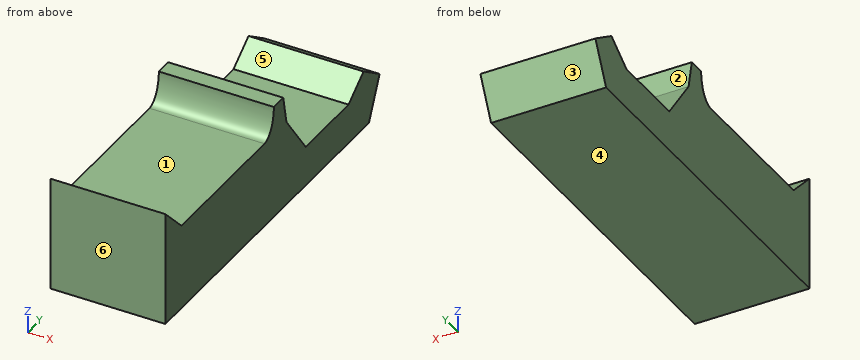
```python
from build123d import *

# Parameters (mm, degrees)
ESQUISSE1_W                   = 600
ESQUISSE1_H                   = 600
BOSS_EXTRU_1_DEPTH            = 2000
ESQUISSE11_W                  = 150
ESQUISSE11_H                  = 800
ENL_V_MAT_EXTRU_1_DEPTH       = 600
ESQUISSE12_W                  = 150
ESQUISSE12_H                  = 1100
ENL_V_MAT_EXTRU_2_DEPTH       = 600
ESQUISSE14_W                  = 150
ESQUISSE14_H                  = 150
BOSS_EXTRU_3_DEPTH            = 600
ENL_V_MAT_EXTRU_5_DEPTH       = 600
ESQUISSE19_W                  = 150
ESQUISSE19_H                  = 100
ENL_V_MAT_EXTRU_6_DEPTH       = 600
ESQUISSE25_W                  = 150
ESQUISSE25_H                  = 100
BOSS_EXTRU_4_DEPTH            = 600
ESQUISSE26_W                  = 150
ESQUISSE26_H                  = 75
BOSS_EXTRU_7_DEPTH            = 600
ESQUISSE30_RX                 = 150
ESQUISSE30_RY                 = 87.5
ENL_V_MAT_EXTRU_7_DEPTH       = 600
ESQUISSE32_W                  = 150
ESQUISSE32_H                  = 30
BOSS_EXTRU_8_DEPTH            = 600
ENL_V_MAT_EXTRU_8_DEPTH       = 2158.978826807
ENL_V_MAT_EXTRU_8_DEPTH_BACK  = 600
ESQUISSE34_W                  = 240
ESQUISSE34_H                  = 870
ENL_V_MAT_EXTRU_9_DEPTH       = 600
ESQUISSE35_W                  = 240
ESQUISSE35_H                  = 180
BOSS_EXTRU_9_DEPTH            = 600
ENL_V_START                   = -600
ENL_V_MAT_EXTRU_10_DEPTH      = 600
ENL_V_MAT_EXTRU_11_DEPTH      = 2158.978826807
ENL_V_MAT_EXTRU_11_DEPTH_BACK = 600
ENL_V_MAT_EXTRU_12_DEPTH      = 2158.978826807
ENL_V_MAT_EXTRU_12_DEPTH_BACK = 600
ESQUISSE41_W                  = 210
ESQUISSE41_H                  = 100
BOSS_EXTRU_10_DEPTH           = 600
ESQUISSE43_W                  = 100
ESQUISSE43_H                  = 150
BOSS_EXTRU_12_DEPTH           = 600
ESQUISSE44_W                  = 100
ESQUISSE44_H                  = 140
BOSS_EXTRU_13_DEPTH           = 600
ENL_V_MAT_EXTRU_13_DEPTH      = 600
ENL_V_MAT_EXTRU_14_DEPTH      = 600
ENL_V_MAT_EXTRU_15_DEPTH      = 600


# Read off the part's stored shape, not the designer's step: Enlèv. mat.-Extru.10
with BuildPart() as part:
    # Esquisse1 → Boss.-Extru.1 (new body)
    with BuildSketch(Plane(origin=(0, 0, 0), x_dir=(1, 0, 0), z_dir=(0, 1, 0))):
        with Locations((224.80933771, 244.860180987)):
            Rectangle(ESQUISSE1_W, ESQUISSE1_H)
    extrude(amount=BOSS_EXTRU_1_DEPTH)

    # Esquisse11 → Enlèv. mat.-Extru.1 (cut)
    with BuildSketch(Plane(origin=(524.80933771, 0, 0), x_dir=(0, 0, -1), z_dir=(1, 0, 0))):
        with Locations((19.860180987, 400)):
            Rectangle(ESQUISSE11_W, ESQUISSE11_H)
    extrude(amount=-ENL_V_MAT_EXTRU_1_DEPTH, mode=Mode.SUBTRACT)

    # Esquisse12 → Enlèv. mat.-Extru.2 (cut)
    with BuildSketch(Plane(origin=(524.80933771, 0, 0), x_dir=(0, 0, -1), z_dir=(1, 0, 0))):
        with Locations((19.860180987, 1450)):
            Rectangle(ESQUISSE12_W, ESQUISSE12_H)
    extrude(amount=-ENL_V_MAT_EXTRU_2_DEPTH, mode=Mode.SUBTRACT)

    # Esquisse14 → Boss.-Extru.3 (add)
    with BuildSketch(Plane(origin=(524.80933771, 0, 0), x_dir=(0, 0, -1), z_dir=(1, 0, 0))):
        with Locations((19.860180987, 75)):
            Rectangle(ESQUISSE14_W, ESQUISSE14_H)
    extrude(amount=-BOSS_EXTRU_3_DEPTH)

    # Esquisse18 → Enlèv. mat.-Extru.5 (cut)
    with BuildSketch(Plane(origin=(524.80933771, 0, 0), x_dir=(0, 0, -1), z_dir=(1, 0, 0))):
        Polygon((94.860180987, 150), (-55.139819013, 0), (-55.139819013, 150), align=None)
    extrude(amount=-ENL_V_MAT_EXTRU_5_DEPTH, mode=Mode.SUBTRACT)

    # Esquisse19 → Enlèv. mat.-Extru.6 (cut)
    with BuildSketch(Plane(origin=(524.80933771, 0, 0), x_dir=(0, 0, -1), z_dir=(1, 0, 0))):
        with Locations((19.860180987, 850)):
            Rectangle(ESQUISSE19_W, ESQUISSE19_H)
    extrude(amount=-ENL_V_MAT_EXTRU_6_DEPTH, mode=Mode.SUBTRACT)

    # Esquisse25 → Boss.-Extru.4 (add)
    with BuildSketch(Plane(origin=(524.80933771, 0, 0), x_dir=(0, 0, -1), z_dir=(1, 0, 0))):
        with Locations((19.860180987, 1050)):
            Rectangle(ESQUISSE25_W, ESQUISSE25_H)
    extrude(amount=-BOSS_EXTRU_4_DEPTH)

    # Esquisse26 → Boss.-Extru.7 (add)
    with BuildSketch(Plane(origin=(524.80933771, 0, 0), x_dir=(0, 0, -1), z_dir=(1, 0, 0))):
        with Locations((19.860180987, 962.5)):
            Rectangle(ESQUISSE26_W, ESQUISSE26_H)
    extrude(amount=-BOSS_EXTRU_7_DEPTH)

    # Esquisse30 → Enlèv. mat.-Extru.7 (cut)
    with BuildSketch(Plane(origin=(524.80933771, 0, 0), x_dir=(0, 0, -1), z_dir=(1, 0, 0))):
        with Locations((-55.139819013, 925)):
            Ellipse(ESQUISSE30_RX, ESQUISSE30_RY)
    extrude(amount=-ENL_V_MAT_EXTRU_7_DEPTH, mode=Mode.SUBTRACT)

    # Esquisse32 → Boss.-Extru.8 (add)
    with BuildSketch(Plane(origin=(524.80933771, 0, 0), x_dir=(0, 0, -1), z_dir=(1, 0, 0))):
        with Locations((19.860180987, 1115)):
            Rectangle(ESQUISSE32_W, ESQUISSE32_H)
    extrude(amount=-BOSS_EXTRU_8_DEPTH)

    # Esquisse33 → Enlèv. mat.-Extru.8 (cut, two sides: drawn at the far end of the back side and taken through both)
    with BuildSketch(Plane(origin=(524.80933771, 0, 0), x_dir=(0, 0, -1), z_dir=(1, 0, 0)).offset(-ENL_V_MAT_EXTRU_8_DEPTH_BACK)):
        Polygon((94.860180987, 1130), (-55.139819013, 1130), (-55.139819013, 1100), align=None)
    extrude(amount=ENL_V_MAT_EXTRU_8_DEPTH + ENL_V_MAT_EXTRU_8_DEPTH_BACK, mode=Mode.SUBTRACT)

    # Esquisse34 → Enlèv. mat.-Extru.9 (cut)
    with BuildSketch(Plane(origin=(524.80933771, 0, 0), x_dir=(0, 0, -1), z_dir=(1, 0, 0))):
        with Locations((214.860180987, 1565)):
            Rectangle(ESQUISSE34_W, ESQUISSE34_H)
    extrude(amount=-ENL_V_MAT_EXTRU_9_DEPTH, mode=Mode.SUBTRACT)

    # Esquisse35 → Boss.-Extru.9 (add)
    with BuildSketch(Plane(origin=(524.80933771, 0, 0), x_dir=(0, 0, -1), z_dir=(1, 0, 0))):
        with Locations((214.860180987, 1220)):
            Rectangle(ESQUISSE35_W, ESQUISSE35_H)
    extrude(amount=-BOSS_EXTRU_9_DEPTH)

    # Enlèv. mat.-Extru.10 outline → Enlèv. mat.-Extru.10 (cut)
    with BuildSketch(Plane(origin=(524.80933771, 0, 0), x_dir=(0, 0, -1), z_dir=(1, 0, 0)).offset(ENL_V_START)):
        Polygon((94.860180987, 1310), (94.860180987, 1130), (334.860180987, 1310), align=None)
    extrude(amount=ENL_V_MAT_EXTRU_10_DEPTH, mode=Mode.SUBTRACT)

    # Esquisse37 → Enlèv. mat.-Extru.11 (cut, two sides: drawn at the far end of the back side and taken through both)
    with BuildSketch(Plane(origin=(524.80933771, 0, 0), x_dir=(0, 0, -1), z_dir=(1, 0, 0)).offset(-ENL_V_MAT_EXTRU_11_DEPTH_BACK)):
        Polygon((544.860180987, 1900), (544.860180987, 2000), (394.860180987, 2000), align=None)
    extrude(amount=ENL_V_MAT_EXTRU_11_DEPTH + ENL_V_MAT_EXTRU_11_DEPTH_BACK, mode=Mode.SUBTRACT)

    # Esquisse38 → Enlèv. mat.-Extru.12 (cut, two sides: drawn at the far end of the back side and taken through both)
    with BuildSketch(Plane(origin=(524.80933771, 0, 0), x_dir=(0, 0, -1), z_dir=(1, 0, 0)).offset(-ENL_V_MAT_EXTRU_12_DEPTH_BACK)):
        Polygon((2509.437735817, 5524.295924716), (394.860180987, 2000), (334.860180987, 1900), (-1779.717373842, -1624.295924716), (-8828.309223275, 2604.859184943), (-4539.154113615, 9753.451034376), align=None)
    extrude(amount=ENL_V_MAT_EXTRU_12_DEPTH + ENL_V_MAT_EXTRU_12_DEPTH_BACK, mode=Mode.SUBTRACT)

    # Esquisse41 → Boss.-Extru.10 (add)
    with BuildSketch(Plane(origin=(524.80933771, 0, 0), x_dir=(0, 0, -1), z_dir=(1, 0, 0))):
        with Locations((439.860180987, 1950)):
            Rectangle(ESQUISSE41_W, ESQUISSE41_H)
    extrude(amount=-BOSS_EXTRU_10_DEPTH)

    # Esquisse43 → Boss.-Extru.12 (add)
    with BuildSketch(Plane(origin=(524.80933771, 0, 0), x_dir=(0, 0, -1), z_dir=(1, 0, 0))):
        with Locations((284.860180987, 1925)):
            Rectangle(ESQUISSE43_W, ESQUISSE43_H)
    extrude(amount=-BOSS_EXTRU_12_DEPTH)

    # Esquisse44 → Boss.-Extru.13 (add)
    with BuildSketch(Plane(origin=(524.80933771, 0, 0), x_dir=(0, 0, -1), z_dir=(1, 0, 0))):
        with Locations((284.860180987, 1780)):
            Rectangle(ESQUISSE44_W, ESQUISSE44_H)
    extrude(amount=-BOSS_EXTRU_13_DEPTH)

    # Esquisse45 → Enlèv. mat.-Extru.13 (cut)
    with BuildSketch(Plane(origin=(524.80933771, 0, 0), x_dir=(0, 0, -1), z_dir=(1, 0, 0))):
        Polygon((334.860180987, 1710), (234.860180987, 1850), (234.860180987, 1710), align=None)
    extrude(amount=-ENL_V_MAT_EXTRU_13_DEPTH, mode=Mode.SUBTRACT)

    # Esquisse46 → Enlèv. mat.-Extru.14 (cut)
    with BuildSketch(Plane(origin=(524.80933771, 0, 0), x_dir=(0, 0, -1), z_dir=(1, 0, 0))):
        Polygon((234.860180987, 1850), (334.860180987, 2000), (234.860180987, 2000), align=None)
    extrude(amount=-ENL_V_MAT_EXTRU_14_DEPTH, mode=Mode.SUBTRACT)

    # Esquisse47 → Enlèv. mat.-Extru.15 (cut)
    with BuildSketch(Plane(origin=(524.80933771, 0, 0), x_dir=(0, 0, -1), z_dir=(1, 0, 0))):
        Polygon((544.860180987, 2000), (334.860180987, 2000), (544.860180987, 1900), align=None)
    extrude(amount=-ENL_V_MAT_EXTRU_15_DEPTH, mode=Mode.SUBTRACT)


solid = part.part
```
For this review, take the finished solid that the model builds, in its own axes (mm). Face numbers are marked on the shaded views. A direction names the side the tool comes from. Round coordinates to 2 decimals unless told otherwise and drop trailing zeros. Write each loop counter-clockwise with the first axis right and the second up, starting at its lowest first coordinate (ties: lowest second). Pieces come first, ordered by that corner, then holes. Notation, with made-up numbers: (69.25, -19.75) -> (128.25, -19.75) arc R16 cw to (128.25, 6.25) -> close; hole circle Ø4 at (-5, 7). An arc over 180 degrees is marked (long way). One line per question, with ' | ' between items. Start each with the question number.
(1) Mouldability with a two-part tool opening along Y and no side actions: class the marked faces 3, 4, 5 and 6 as released by +Y, released by -Y, zero draft, split by the parting line, or undercut.
(2) Add section B-B, the plane z = -197. Write out the cut boundary in (x, y), plus the area to 3 significant figures.
(3) Add section A-A, the plane y = 572.5. Write out the cut boundary in (x, z).
(4) For line 1 along Z through (x, y) = (327.5, 870.5); line 2 along Y through (x, z) = (222.5, -66); line 3 along Y through (x, z) = (242, -282), list the stretches that pass through material, from the lowest coordinate up. Write a range as from..to.
(5) Tool access review of the marked faces 1 and 2: name each direction out of +Z, -Z, +X, -X, +Y, -Y from which nothing blocks a thin tool from reaching the whole face with its end or side.
(6) Insertion check: P1, Ø6, axis at x = 167, y = 788, coming from the +Z side; P2, Ø12, axis at x = 46.5, z = -355, coming from the +Y side; P3, Ø6, axis at x = 64, z = -454, coming from the +Y side. Each pin has a flat end and moves straight along its axis. Give the tip position at first contact, or say it passes through.
Answer list:
1) face 3: released by +Y | face 4: zero draft | face 5: undercut | face 6: released by -Y
2) outline: (-75.19, 0) -> (524.81, 0) -> (524.81, 1206.6) -> (-75.19, 1206.6) -> close | area: 724,000 mm²
3) outline: (-75.19, -544.86) -> (524.81, -544.86) -> (524.81, -94.86) -> (-75.19, -94.86) -> close
4) line 1: -544.86..-94.86 | line 2: 0..121.14, 976.6..1124.23 | line 3: 0..1270.35, 1784..1920.71
5) face 1: +Z, +X, -X | face 2: +Z, +X, -X, +Y
6) P1: z = -94.86 | P2: y = 1993.27 | P3: y = 1944.7
